Part model, mm, in its own coordinate system. Coordinates: 2 decimals unless noted, no trailing zeros. Write each loop counter-clockwise with the first axis right and the second up, starting at its lowest first coordinate (ties: lowest second). Pieces come first, ordered by that corner, then holes. Notation, with made-up numbers: (-22.5, -30.75) - (32.5, -30.75) arc R21 cw to (32.5, 6.25) - close; hole circle Ø11 at (59.25, -25). An arc over 180 degrees is marked (long way). Write each question's results on one line, items separated by ' | '.
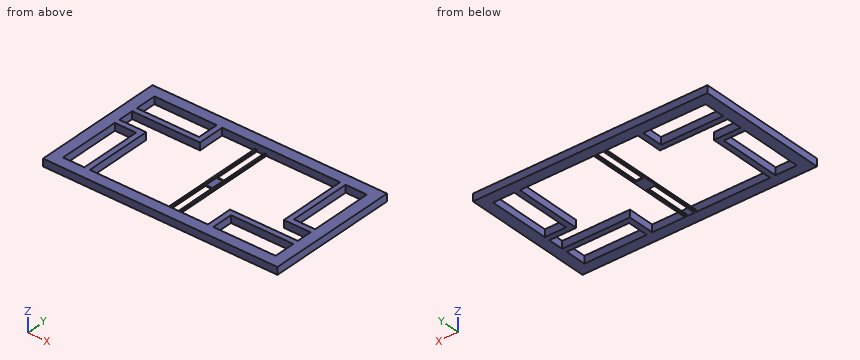
from build123d import *

# Parameters (mm, degrees)
ESBO_O1_W                = 640
ESBO_O1_H                = 360
ESBO_O1_W_2              = 170
ESBO_O1_H_2              = 58
ESBO_O1_W_3              = 58
ESBO_O1_H_3              = 170
RESSALTO_EXTRUS_O1_DEPTH = 20
SKETCH1_W                = 5
SKETCH1_H                = 5
BOSS_EXTRUDE1_DEPTH      = 300
SKETCH2_W                = 2
SKETCH2_H                = 34
BOSS_EXTRUDE2_DEPTH      = 21
SKETCH3_W                = 3
SKETCH3_H                = 2
BOSS_EXTRUDE3_DEPTH      = 21


with BuildPart() as part:
    # Esboço1 → Ressalto-extrusão1 (new body)
    with BuildSketch(Plane.XY):
        with Locations((320, 180)):
            Rectangle(ESBO_O1_W, ESBO_O1_H)
        Polygon((215, 330), (537, 330), (537, 160), (537, 145), (610, 145), (610, 103), (425, 103), (425, 88), (425, 30), (103, 30), (103, 215), (88, 215), (30, 215), (30, 257), (200, 257), (215, 257), align=None, mode=Mode.SUBTRACT)
        with Locations((115, 301)):
            Rectangle(ESBO_O1_W_2, ESBO_O1_H_2, mode=Mode.SUBTRACT)
        with Locations((59, 115)):
            Rectangle(ESBO_O1_W_3, ESBO_O1_H_3, mode=Mode.SUBTRACT)
        with Locations((581, 245)):
            Rectangle(ESBO_O1_W_3, ESBO_O1_H_3, mode=Mode.SUBTRACT)
        with Locations((525, 59)):
            Rectangle(ESBO_O1_W_2, ESBO_O1_H_2, mode=Mode.SUBTRACT)
    extrude(amount=RESSALTO_EXTRUS_O1_DEPTH)

    # Sketch1 → Boss-Extrude1 (add)
    with BuildSketch(Plane.XZ.offset(-330)):
        with Locations((307, 2.5)):
            Rectangle(SKETCH1_W, SKETCH1_H)
        with Locations((333, 2.5)):
            Rectangle(SKETCH1_W, SKETCH1_H)
    extrude(amount=BOSS_EXTRUDE1_DEPTH)

    # Sketch2 → Boss-Extrude2 (add)
    with BuildSketch(Plane(origin=(309.5, 0, 0), x_dir=(0, 0, -1), z_dir=(1, 0, 0))):
        with Locations((-1, 180)):
            Rectangle(SKETCH2_W, SKETCH2_H)
    extrude(amount=BOSS_EXTRUDE2_DEPTH)

    # Sketch3 → Boss-Extrude3 (add)
    with BuildSketch(Plane(origin=(309.5, 0, 0), x_dir=(0, 0, -1), z_dir=(1, 0, 0))):
        with Locations((-1.5, 198)):
            Rectangle(SKETCH3_W, SKETCH3_H)
        with Locations((-1.5, 162)):
            Rectangle(SKETCH3_W, SKETCH3_H)
    extrude(amount=BOSS_EXTRUDE3_DEPTH)


solid = part.part
(1) Flat gauge pins, fed straight in: P1, Ø1.6, axis at x = 321, y = 161.5, coming from the +Z side; P2, Ø4, axis at x = 307, y = 164, coming from the +Z side. Where does each tip first touch, or does it go through?
Return value:
P1: stops at z = 3 | P2: stops at z = 5
(2) Wall check: line 1 (Y direction, x = 67, z = 15); line 2 (Y direction, x = 464, z = 8.5); line 3 (X direction, y = 294.5, z = 2.5). Give the ranges that are in metal, low to high. Write a range as from..to.
Return value:
line 1: y = 0..30, 200..215, 257..272, 330..360 | line 2: y = 0..30, 88..103, 330..360 | line 3: x = 0..30, 200..215, 304.5..309.5, 330.5..335.5, 537..552, 610..640
(3) Saw through at B-B on x = 481. Write the cut outline in (y, z).
Return value:
outline: (0, 0) - (30, 0) - (30, 20) - (0, 20) - close; (88, 0) - (103, 0) - (103, 20) - (88, 20) - close; (330, 0) - (360, 0) - (360, 20) - (330, 20) - close
(4) Saw through at D-D on x = 568.5. Write the cut outline in (y, z).
Return value:
outline: (0, 0) - (30, 0) - (30, 20) - (0, 20) - close; (88, 0) - (103, 0) - (103, 20) - (88, 20) - close; (145, 0) - (160, 0) - (160, 20) - (145, 20) - close; (330, 0) - (360, 0) - (360, 20) - (330, 20) - close
(5) Saw through at A-A on y = 135. Write the cut outline in (x, z).
Return value:
outline: (0, 0) - (30, 0) - (30, 20) - (0, 20) - close; (88, 0) - (103, 0) - (103, 20) - (88, 20) - close; (304.5, 0) - (309.5, 0) - (309.5, 5) - (304.5, 5) - close; (330.5, 0) - (335.5, 0) - (335.5, 5) - (330.5, 5) - close; (610, 0) - (640, 0) - (640, 20) - (610, 20) - close
(6) Saw through at C-C on z = 12. Count the separate pieces of the cut face and the enclosed holes in it, then the cut area to 3 significant figures.
Return value:
separate pieces: 1 | enclosed holes: 5 | area: 71,000 mm^2
